Can you work these out from the model? Positions are in its coordinate system, mm. A direction names the side the tool comes from. Give positions to 0.01 mm unless a question says otherwise; leave off trailing zeros. Order: outer loops, then holes, each group sorted by start corner. A loop starts at its lowest first (then second) coordinate and runs counter-clockwise, first axis right, second up. Notation, with made-up numbers: (19.25, 17.25) -> (76.25, 17.25) arc R8 cw to (76.25, 26.25) -> close; hole circle Ø1 at (56.25, 39). An arc over 180 degrees is marked (long way). Answer as a JSON object with one key per item and string values.
```python
from build123d import *

# Parameters (mm, degrees)
SKETCH1_W      = 22.5
SKETCH1_H      = 12
EXTRUDE1_DEPTH = 18
SKETCH2_W      = 32.5
SKETCH2_H      = 12
EXTRUDE2_DEPTH = 2
SKETCH3_W      = 22.5
SKETCH3_H      = 12
EXTRUDE3_DEPTH = 4
SKETCH4_R      = 1
EXTRUDE4_DEPTH = 21
EXTRUDE5_DEPTH = 4.5
SKETCH6_R      = 2.25
EXTRUDE6_DEPTH = 4


with BuildPart() as part:
    # Sketch1 → Extrude1 (new body)
    with BuildSketch(Plane.XY):
        Rectangle(SKETCH1_W, SKETCH1_H)
    extrude(amount=EXTRUDE1_DEPTH)

    # Sketch2 → Extrude2 (add)
    with BuildSketch(Plane.XY.offset(18)):
        Rectangle(SKETCH2_W, SKETCH2_H)
    extrude(amount=EXTRUDE2_DEPTH)

    # Sketch3 → Extrude3 (add)
    with BuildSketch(Plane.XY.offset(20)):
        Rectangle(SKETCH3_W, SKETCH3_H)
    extrude(amount=EXTRUDE3_DEPTH)

    # Sketch4 → Extrude4 (cut, through all)
    with BuildSketch(Plane.XY.offset(20)):
        with Locations((-13.75, 0)):
            Circle(SKETCH4_R)
        with Locations((13.75, 0)):
            Circle(SKETCH4_R)
    extrude(amount=-EXTRUDE4_DEPTH, mode=Mode.SUBTRACT)

    # Sketch5 → Extrude5 (add)
    with BuildSketch(Plane.XY.offset(24)):
        with BuildLine():
            ThreePointArc((-0.229166667, -2.445144707), (11.25, 0), (-0.229166667, 2.445144707))
            ThreePointArc((-0.229166667, 2.445144707), (-3.25, 0), (-0.229166667, -2.445144707))
        make_face()
    extrude(amount=EXTRUDE5_DEPTH)

    # Sketch6 → Extrude6 (add)
    with BuildSketch(Plane.XY.offset(28.5)):
        with Locations((5.25, 0)):
            Circle(SKETCH6_R)
    extrude(amount=EXTRUDE6_DEPTH)


solid = part.part
```
1. If we section it at B-B on z = 19: Please give me the cut outline in (x, y), then the cut area to 3 significant figures.
Worked answers:
{"outline": "(-16.25, -6) -> (16.25, -6) -> (16.25, 6) -> (-16.25, 6) -> close; hole circle Ø2 at (-13.75, 0); hole circle Ø2 at (13.75, 0)", "area": "384 mm²"}
2. Will these pins go through, and if not, where does the flat tip stop? pin 1 Ø3 at (y, z) = (-1, 23) entering from -X; pin 2 Ø1.5 at (x, y) = (-14.5, -2) entering from -Z; pin 3 Ø4 at (x, y) = (-12.5, 2) entering from +Z.
Worked answers:
{"pin 1": "x = -11.25", "pin 2": "z = 18", "pin 3": "z = 24"}
3. If we section it at A-A on x = 13.75: Please give me the cut outline in (y, z).
Worked answers:
{"outline": "(-6, 18) -> (-1, 18) -> (-1, 20) -> (-6, 20) -> close; (1, 18) -> (6, 18) -> (6, 20) -> (1, 20) -> close"}
4. Please list where these lines run through material, in increasing order: L1, parallel to Y at x = 13.75, z = 19.1; L2, parallel to Z at x = 8.5, y = 2.5; L3, parallel to X at y = -4.75, z = 20.5.
Worked answers:
{"L1": "-6 to -1, 1 to 6", "L2": "0 to 28.5", "L3": "-11.25 to 11.25"}
5. For faces 1 (the face through (-15, 0, 18)), 2 (the face through (2, 0, 28.5)), 3 (the face through (-11.25, 0, 22)), 4 (the face through (10, -5, 24)), which set-ups out of +Z, -Z, +X, -X, +Y, -Y let a thin tool reach every point of the face, with its end or its side?
Worked answers:
{"face 1": "-Z, -X, +Y, -Y", "face 2": "+Z", "face 3": "+Z, -X, +Y, -Y", "face 4": "+Z, +X, -Y"}
6. If we section it at C-C on x = -0.75: Please give me the cut outline in (y, z).
Worked answers:
{"outline": "(-6, 0) -> (6, 0) -> (6, 24) -> (2.5, 24) -> (2.5, 28.5) -> (-2.5, 28.5) -> (-2.5, 24) -> (-6, 24) -> close"}
7. If we section it at D-D on z = 29: Please give me the cut outline in (x, y).
Worked answers:
{"outline": "circle Ø4.5 at (5.25, 0)"}
